Could you check a few things on this model? Use its own coordinates, in mm. Round coordinates to 2 decimals unless told otherwise and drop trailing zeros. Loops run counter-clockwise (first coordinate to the right, second up) from the corner with the lowest first, then second, coordinate; pieces in that order, holes last. Notation, with made-up numbers: M -27,40 L 24,40 A20 ccw 24,52 Z; hole C -37.5,74 d1. An arc over 180 degrees is marked long. Return JSON: item names as keys, results as strings. Group by question number.
```python
from build123d import *

# Parameters (mm, degrees)
CROQUIS1_W              = 30
CROQUIS1_H              = 25
SALIENTE_EXTRUIR1_DEPTH = 24
CROQUIS2_R              = 7.5
CORTAR_EXTRUIR1_DEPTH   = 24
CORTAR_EXTRUIR4_REACH   = 41.639
CROQUIS4_R              = 2.25


with BuildPart() as part:
    # Croquis1 → Saliente-Extruir1 (new body)
    with BuildSketch(Plane(origin=(0, 0, 0), x_dir=(0, 0, -1), z_dir=(1, 0, 0))):
        with Locations((4.241023359, 4.022714127)):
            Rectangle(CROQUIS1_W, CROQUIS1_H)
    extrude(amount=SALIENTE_EXTRUIR1_DEPTH)

    # Croquis2 → Cortar-Extruir1 (cut)
    with BuildSketch(Plane.ZY):
        with Locations((-4.241023359, 4.022714127)):
            Circle(CROQUIS2_R)
    extrude(amount=-CORTAR_EXTRUIR1_DEPTH, mode=Mode.SUBTRACT)

    # Croquis4 → Cortar-Extruir4 (cut, up to next)
    with BuildSketch(Plane(origin=(0, 16.522714127, 0), x_dir=(1, 0, 0), z_dir=(0, 1, 0)), mode=Mode.PRIVATE) as cortar_extruir4_sk1:
        with Locations(Location((12, 15.491023359, 0), (0, 0, 270))):
            Circle(CROQUIS4_R)
    cortar_extruir4_tool1 = extrude(cortar_extruir4_sk1.sketch, amount=-CORTAR_EXTRUIR4_REACH, mode=Mode.PRIVATE) & part.part
    # Croquis4 → Cortar-Extruir4 (cut, up to next)
    with BuildSketch(Plane(origin=(0, 16.522714127, 0), x_dir=(1, 0, 0), z_dir=(0, 1, 0)), mode=Mode.PRIVATE) as cortar_extruir4_sk2:
        with Locations(Location((12, -7.008976641, 0), (0, 0, 270))):
            Circle(CROQUIS4_R)
    cortar_extruir4_tool2 = extrude(cortar_extruir4_sk2.sketch, amount=-CORTAR_EXTRUIR4_REACH, mode=Mode.PRIVATE) & part.part
    add(cortar_extruir4_tool1.solids().sort_by_distance((12, 16.522714, -15.491023))[0], mode=Mode.SUBTRACT)
    add(cortar_extruir4_tool2.solids().sort_by_distance((12, 16.522714, 7.008977))[0], mode=Mode.SUBTRACT)


solid = part.part
```
1. I'm going to push a flat-ended pin straight in: pin 1 Ø3.5 at (x, z) = (12, -15.49) entering from -Y. Where does the tip first touch, or does it pass through?
2. If we section it at B-B, the plane y = 8: Please give me the cut outline in (x, z).
3. If we section it at C-C, the plane z = -7.5: Please give me the cut outline in (x, y), then the cut area to 3 significant figures.
4. We'd pull the mould along Z, two halves only. Please class faces 1 (the face through (13.52, 4.2, 5.35)), 2 (the face through (11.832, -0.541, -10.193)), 3 (the face through (0, 13, -4)), 4 (the face through (12, 4, 10.759)): +Z half, -Z half, draft (parallel to the pull), parting line (faces both ways), or undercut.
5. If we section it at A-A, the plane x = 13.5: Please give me the cut outline in (y, z).
6. I need wall thicknesses on probe 1 along Z at (x, y) = (6.5, 4.25); probe 2 along Z at (x, y) = (10.25, 0.5); probe 3 along Y at (x, z) = (3, 2.25). Which ranges of each line are inside material? Lowest first, please.
7. If we section it at D-D, the plane y = 4.5: Please give me the cut outline in (x, z), then the cut area to 3 significant figures.
Geometry results:
{
 "1": {"pin 1": "through"},
 "2": {"outline": "M 0,-19.24 L 24,-19.24 L 24,-10.6 L 0,-10.6 Z; M 0,2.12 L 24,2.12 L 24,10.76 L 0,10.76 Z; hole C 12,-15.49 d4.5; hole C 12,7.01 d4.5"},
 "3": {"outline": "M 0,-8.48 L 24,-8.48 L 24,-2.73 L 0,-2.73 Z; M 0,10.78 L 24,10.78 L 24,16.52 L 0,16.52 Z", "area": "276 mm^2"},
 "4": {"face 1": "undercut", "face 2": "undercut", "face 3": "draft", "face 4": "+Z half"},
 "5": {"outline": "M -8.48,-19.24 L 16.52,-19.24 L 16.52,-17.17 L -8.48,-17.17 Z; M -8.48,-13.81 L 16.52,-13.81 L 16.52,5.33 L -8.48,5.33 Z; M -8.48,8.69 L 16.52,8.69 L 16.52,10.76 L -8.48,10.76 Z; hole C 4.02,-4.24 d15"},
 "6": {"probe 1": "-19.24 to -11.74, 3.26 to 10.76", "probe 2": "-19.24 to -16.91, -14.08 to -10.86, 2.38 to 5.59, 8.42 to 10.76", "probe 3": "-8.48 to 0.27, 7.78 to 16.52"},
 "7": {"outline": "M 0,-19.24 L 24,-19.24 L 24,-11.73 L 0,-11.73 Z; M 0,3.24 L 24,3.24 L 24,10.76 L 0,10.76 Z; hole C 12,-15.49 d4.5; hole C 12,7.01 d4.5", "area": "329 mm^2"}
}
